The listing builds one solid part. Answer for the finished solid, in the listing's coordinates (mm). Give positions to 0.01 mm unless a question says otherwise; leave off trailing zeros. Order: outer loops, then holes, each group sorted by start corner. A loop starts at its lowest first (then second) coordinate and runs counter-clockwise, first axis right, second up. Notation, with made-up numbers: (24, -27) - (67, -27) arc R20 cw to (67, -14) - close; hole circle Ø7 at (-4.5, 41.5). An arc over 180 degrees is marked (long way). Answer in a Markdown table with one row per item.
from build123d import *

# Parameters (mm, degrees)
F0_R          = 7.1
F1_DEPTH      = 60
F2_W          = 30
F2_H          = 27.0439040799
F3_DEPTH      = 25
F3_DEPTH_BACK = 25


with BuildPart() as f1:
    # F0 (on Front) → F1 (new body)
    with BuildSketch(Plane.XZ):
        with BuildLine():
            Line((-10.5591211108, 319.1935136895), (-10.5583761074, 9.1935136904))
            ThreePointArc((-10.5583761074, 9.1935136904), (-0.0005672768, -13.9999999885), (10.5591211108, 9.1926580142))
            Line((10.5591211108, 9.1926580142), (10.5583761074, 319.1926580133))
            Line((10.5583761074, 319.1926580133), (-10.5591211108, 319.1935136895))
        make_face()
        Circle(F0_R, mode=Mode.SUBTRACT)
    extrude(amount=F1_DEPTH)

    # F2 (on Right) → F3 (cut, two sides)
    with BuildSketch(Plane.YZ) as f3_sk:
        with Locations((-30, -1.146184979)):
            Rectangle(F2_W, F2_H)
    extrude(amount=-F3_DEPTH, mode=Mode.SUBTRACT)
    extrude(f3_sk.sketch, amount=F3_DEPTH_BACK, mode=Mode.SUBTRACT)


solid = f1.part
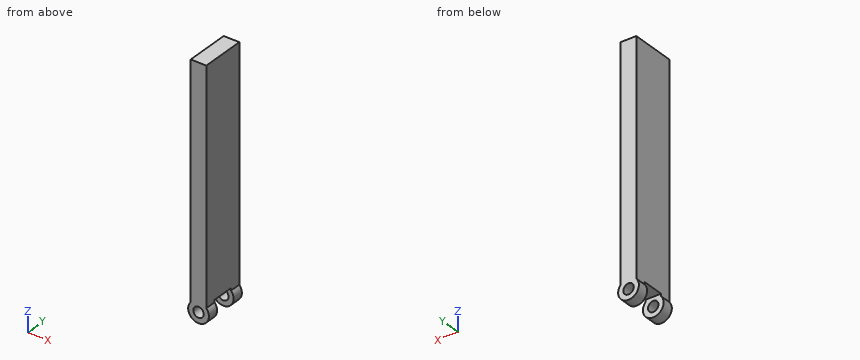
Item 1: Find section D-D on y = -18. Write down the section's boundary in (x, z), then the cut area to 3 significant figures.
Answer block:
| item | result |
|---|---|
| outline | (-10.56, 12.38) - (10.56, 12.38) - (10.56, 319.19) - (-10.56, 319.19) - close |
| area | 6,480 mm² |
Item 2: Consider line 1 (Z direction, x = -0.5, y = -56); line 2 (X direction, y = -8.5, z = 27.5); line 3 (X direction, y = -4.25, z = 0). Determine where each line is inside the solid, lowest interval first.
Answer block:
| item | result |
|---|---|
| line 1 | -13.99 to -7.08, 7.08 to 319.19 |
| line 2 | -10.56 to 10.56 |
| line 3 | -14 to -7.1, 7.1 to 14 |
Item 3: Find section B-B on z = 0. Write down the section's boundary in (x, y), then the cut area to 3 significant figures.
Answer block:
| item | result |
|---|---|
| outline | (-14, -60) - (-7.1, -60) - (-7.1, -45) - (-14, -45) - close; (-14, -15) - (-7.1, -15) - (-7.1, 0) - (-14, 0) - close; (7.1, -60) - (14, -60) - (14, -45) - (7.1, -45) - close; (7.1, -15) - (14, -15) - (14, 0) - (7.1, 0) - close |
| area | 414 mm² |
Item 4: Find section A-A on y = -6. Write down the section's boundary in (x, z).
Answer block:
| item | result |
|---|---|
| outline | (-10.56, 9.19) arc R14 ccw (long way) to (10.56, 9.19) - (10.56, 319.19) - (-10.56, 319.19) - close; hole circle Ø14.2 at (0, 0) |
Item 5: Find section C-C on x = 0. Write down the section's boundary in (y, z).
Answer block:
| item | result |
|---|---|
| outline | (-60, -14) - (-45, -14) - (-45, -7.1) - (-60, -7.1) - close; (-60, 7.1) - (-45, 7.1) - (-45, 12.38) - (-15, 12.38) - (-15, 7.1) - (0, 7.1) - (0, 319.19) - (-60, 319.19) - close; (-15, -14) - (0, -14) - (0, -7.1) - (-15, -7.1) - close |
Item 6: Each of these flat-tipped pins is pushed along its axis until it touches: P1, Ø3, axis at y = -49, z = 176, coming from the -X side; P2, Ø8, axis at x = -8, z = 94.5, coming from the +Y side; P3, Ø5, axis at x = 3.5, y = -18, coming from the -Z side; P4, Ø1, axis at y = -51, z = 216, coming from the +X side. Where does it stop, or does it pass through?
Answer block:
| item | result |
|---|---|
| P1 | x = -10.56 |
| P2 | y = 0 |
| P3 | z = 12.38 |
| P4 | x = 10.56 |
